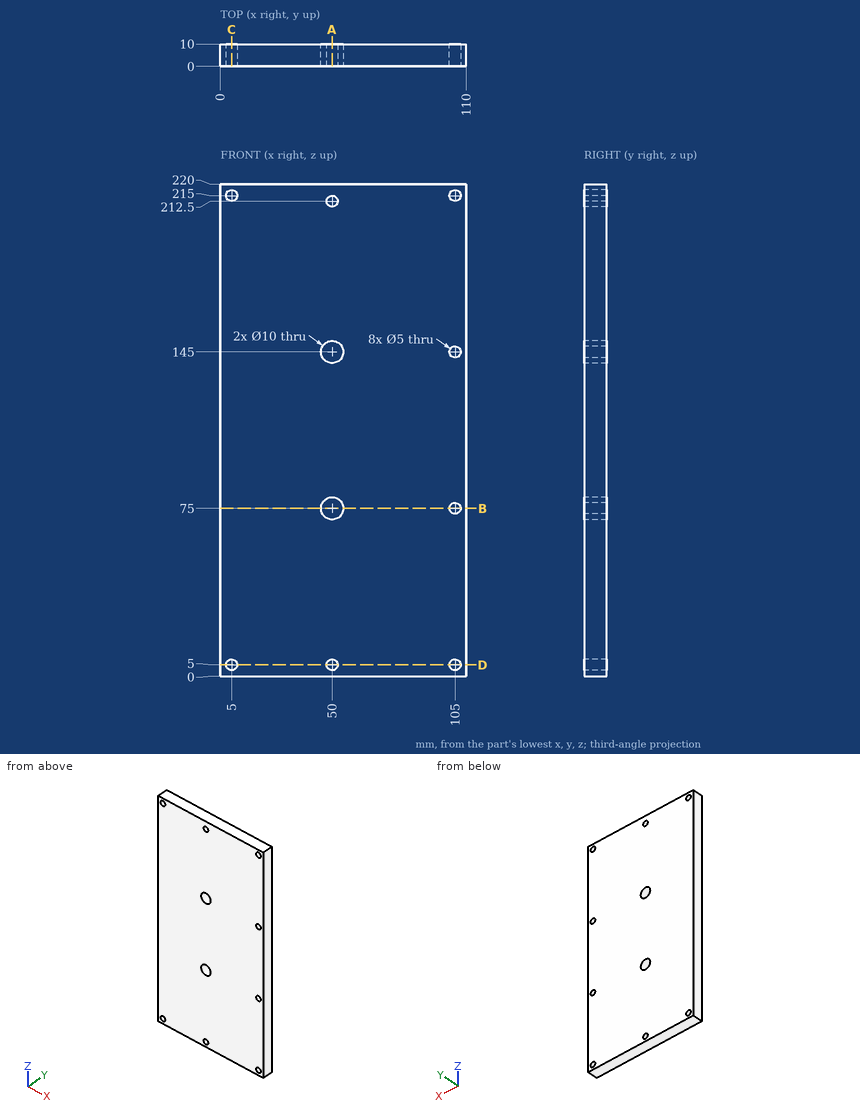
For this review, use the dimensioned drawing (mm, ordinates from the lowest corner) and the shaded views. Round coordinates to 2 decimals unless told otherwise and drop trailing zeros. Write each loop counter-clockwise with the first axis right and the second up, starting at its lowest first coordinate (ties: lowest second). Pieces come first, ordered by that corner, then holes. Notation, with made-up numbers: (36, 79.25) - (74, 79.25) arc R15 ccw to (74, 86.25) - close; hole circle Ø2 at (41, -19.75). An arc over 180 degrees is marked (long way). Use a Markdown table: item, result.
Q1. We need section D-D (z = 5). Give the boundary of the cut face in (x, y), plus the area to 3 significant figures.
Derived:
| item | result |
|---|---|
| outline | (0, 0) - (2.5, 0) - (2.5, 10) - (0, 10) - close; (7.5, 0) - (47.5, 0) - (47.5, 10) - (7.5, 10) - close; (52.5, 0) - (102.5, 0) - (102.5, 10) - (52.5, 10) - close; (107.5, 0) - (110, 0) - (110, 10) - (107.5, 10) - close |
| area | 950 mm2 |
Q2. Clearance check with flat-ended pins moving along their axes: pin 1 (1 mm diameter, centred on y = 6.5, z = 92.5, fed in from -X); pin 2 (4.5 mm diameter, centred on x = 5, z = 215, fed in from +Y). State where each tip first meets the part, or that it passes through.
Derived:
| item | result |
|---|---|
| pin 1 | stops at x = 0 |
| pin 2 | passes through |
Q3. Wall thickness on line 1 along Z through (x, y) = (105, 3.5); line 2 along Z through (x, y) = (49, 4); line 3 along Z through (x, y) = (47, 0.5): over which ranges is each line inside the solid? List them lowest first.
Derived:
| item | result |
|---|---|
| line 1 | z = 0 to 2.5, 7.5 to 72.5, 77.5 to 142.5, 147.5 to 212.5, 217.5 to 220 |
| line 2 | z = 0 to 2.71, 7.29 to 70.1, 79.9 to 140.1, 149.9 to 210.21, 214.79 to 220 |
| line 3 | z = 0 to 71, 79 to 141, 149 to 220 |
Q4. We need section A-A (x = 50). Give the boundary of the cut face in (y, z).
Derived:
| item | result |
|---|---|
| outline | (0, 0) - (10, 0) - (10, 2.5) - (0, 2.5) - close; (0, 7.5) - (10, 7.5) - (10, 70) - (0, 70) - close; (0, 80) - (10, 80) - (10, 140) - (0, 140) - close; (0, 150) - (10, 150) - (10, 210) - (0, 210) - close; (0, 215) - (10, 215) - (10, 220) - (0, 220) - close |
Q5. We need section B-B (z = 75). Give the boundary of the cut face in (x, y), plus the area to 3 significant figures.
Derived:
| item | result |
|---|---|
| outline | (0, 0) - (45, 0) - (45, 10) - (0, 10) - close; (55, 0) - (102.5, 0) - (102.5, 10) - (55, 10) - close; (107.5, 0) - (110, 0) - (110, 10) - (107.5, 10) - close |
| area | 950 mm2 |
Q6. We need section C-C (x = 5). Give the boundary of the cut face in (y, z).
Derived:
| item | result |
|---|---|
| outline | (0, 0) - (10, 0) - (10, 2.5) - (0, 2.5) - close; (0, 7.5) - (10, 7.5) - (10, 212.5) - (0, 212.5) - close; (0, 217.5) - (10, 217.5) - (10, 220) - (0, 220) - close |
